Input: part model. Units: mm. Frame: model coordinates. A direction names the side the tool comes from. Round coordinates to 2 decimals unless told otherwise and drop trailing zeros. Loops run counter-clockwise (first coordinate to the right, second up) from the corner with the lowest first, then second, coordinate; pieces in that order, holes last. Notation, with made-up numbers: M 60.25,48 L 83.25,48 A23 ccw 83.25,60 Z; hole C 86,55 d8. An arc over 180 degrees is marked long. Put each result on its own line as item: value. Start each with the question number.
1) Section A-A on y = 1737. Output: boundary loops of the cut face in (x, z), plus the area to 3 significant figures.
2) Section C-C on y = 341. Output: boundary loops of the cut face in (x, z).
3) Section B-B on x = 6. Output: boundary loops of the cut face in (y, z).
4) Line query: probe 1 along Y at (x, z) = (74.5, 80); probe 2 along Z at (x, y) = (-43, 876.5); probe 3 along Z at (x, y) = (136.5, 1057). Output: solid intervals per line, ascending.
5) Reachability of faces 1 (the face through (2, 1949, 43.132)), 2 (the face through (-2, 986, -21.394)), 3 (the face through (-2, 1300, 68)) from +Z, -Z, +X, -X, +Y, -Y: full face, straight path, thin tool, end or side. Return the list, or none.
6) Section D-D on x = 179. Output: boundary loops of the cut face in (y, z).
7) Draft query along X for faces 4 (the face through (-2, 1600, 68)), 5 (the face through (-2, 1752, 93.132)). Return one class per face: +X half, -X half, draft (parallel to the pull), parting line (faces both ways), or undercut.
8) Pin query (flat end, axial travel): pin 1 (12 mm diameter, centred on x = 36, y = 1569.5, fed in from -Z); pin 2 (1 mm diameter, centred on y = 448, z = 24.5, fed in from -X); pin 3 (5 mm diameter, centred on x = 146.5, y = 1633.5, fed in from +Z). Return the tip coordinate at first contact, or that it passes through.
from build123d import *

# Parameters (mm, degrees)
EXTRUDE_1_DEPTH = 2000
SKETCH_3_W      = 282.482591868
SKETCH_3_H      = 300
EXTRUDE_2_DEPTH = 50


with BuildPart() as part:
    # 草圖2 → 填料-伸長1 (new body)
    with BuildSketch(Plane(origin=(0, 0, 0), x_dir=(1, 0, 0), z_dir=(0, 1, 0))):
        with BuildLine():
            Line((-141.241295934, 21.394189404), (141.241295934, 21.394189404))
            ThreePointArc((141.241295934, 21.394189404), (229.43942383, -10.868839364), (141.241295934, -43.131868132))
            Line((141.241295934, -43.131868132), (-141.241295934, -43.131868132))
            ThreePointArc((-141.241295934, -43.131868132), (-229.43942383, -10.868839364), (-141.241295934, 21.394189404))
        make_face()
    extrude(amount=EXTRUDE_1_DEPTH)

    # 草圖3 → 填料-伸長2 (add)
    with BuildSketch(Plane.XY.offset(43.131868132)):
        with Locations((0, 550)):
            Rectangle(SKETCH_3_W, SKETCH_3_H)
        with Locations((0, 1150)):
            Rectangle(SKETCH_3_W, SKETCH_3_H)
        with Locations((0, 1750)):
            Rectangle(SKETCH_3_W, SKETCH_3_H)
    extrude(amount=EXTRUDE_2_DEPTH)


solid = part.part
Geometry results:
1. outline: M -141.24,-21.39 L 141.24,-21.39 A50 ccw long 141.24,43.13 L 141.24,93.13 L -141.24,93.13 L -141.24,43.13 A50 ccw long Z
1. area: 47,000 mm²
2. outline: M -141.24,-21.39 L 141.24,-21.39 A50 ccw long 141.24,43.13 L -141.24,43.13 A50 ccw long Z
3. outline: M 0,-21.39 L 2000,-21.39 L 2000,43.13 L 1900,43.13 L 1900,93.13 L 1600,93.13 L 1600,43.13 L 1300,43.13 L 1300,93.13 L 1000,93.13 L 1000,43.13 L 700,43.13 L 700,93.13 L 400,93.13 L 400,43.13 L 0,43.13 Z
4. probe 1: y = 400 to 700, 1000 to 1300, 1600 to 1900
4. probe 2: z = -21.39 to 43.13
4. probe 3: z = -21.39 to 93.13
5. face 1: +Z, +Y
5. face 2: -Z, +Y, -Y
5. face 3: +Z
6. outline: M 0,-39.13 L 2000,-39.13 L 2000,60.87 L 0,60.87 Z
7. face 4: undercut
7. face 5: draft
8. pin 1: stops at z = -21.39
8. pin 2: stops at x = -227.68
8. pin 3: stops at z = 50.54
